Verification items for the finished model (mm, model axes). A direction names the side the tool comes from. Coordinates: 2 decimals unless noted, no trailing zeros. Loops run counter-clockwise (first coordinate to the right, second up) from the corner with the lowest first, then second, coordinate; pieces in that order, holes last. Notation, with made-up numbers: (79, 89.5) -> (95, 89.5) arc R19 ccw to (95, 106.5) -> close; hole circle Ø4 at (27, 60.5). An arc over 180 degrees is marked (long way). Write item = value, one per line.
```python
from build123d import *

# Parameters (mm, degrees)
BOSS_EXTRUDE1_DEPTH = 5.2832
SKETCH2_W           = 101.6
SKETCH2_H           = 14.351
BOSS_EXTRUDE2_DEPTH = 5.2832
CHAMFER1_SIZE       = 12.7
CHAMFER1_SIZE_2     = 3.81
CHAMFER2_SIZE       = 12.7
CHAMFER2_SIZE2      = 3.81
CHAMFER3_SIZE       = 3.81
CHAMFER3_SIZE_2     = 12.7


with BuildPart() as part:
    # Sketch1 → Boss-Extrude1 (new body)
    with BuildSketch(Plane(origin=(0, 0, 0), x_dir=(1, 0, 0), z_dir=(0, 1, 0))):
        Polygon((0, 0), (152.4, 0), (144.78, 68.834), (43.18, 68.834), align=None)
    extrude(amount=BOSS_EXTRUDE1_DEPTH)

    # Sketch2 → Boss-Extrude2 (add)
    with BuildSketch(Plane(origin=(0, 0, 0), x_dir=(1, 0, 0), z_dir=(0, 1, 0))):
        with Locations((76.2, -7.1755)):
            Rectangle(SKETCH2_W, SKETCH2_H)
    extrude(amount=BOSS_EXTRUDE2_DEPTH)

    # Chamfer1
    # the kernel refuses this chamfer: 12.7, 3.81 mm, written as the material it takes off along each edge
    with BuildSketch(Plane(origin=(60.699541801, 0, -96.762210753), x_dir=(0.8470671798621036, -0.011069119507992343, 0.531370555633054), z_dir=(-0.5314031118215187, 0, 0.8471190782566561))) as chamfer1_piece_1:
        Polygon((CHAMFER1_SIZE * 0.99993873542, CHAMFER1_SIZE * 0.011069119508), (-CHAMFER1_SIZE_2 * 0.011069119508, CHAMFER1_SIZE_2 * 0.99993873542), (0, 0), align=None)
    extrude(amount=147.193499363, mode=Mode.SUBTRACT)
    with BuildSketch(Plane(origin=(60.699541801, 5.2832, -96.762210753), x_dir=(0.8470671798621036, 0.01106911950799233, 0.531370555633054), z_dir=(-0.5314031118215187, 0, 0.8471190782566561))) as chamfer1_piece_2:
        Polygon((CHAMFER1_SIZE * 0.99993873542, -CHAMFER1_SIZE * 0.011069119508), (-CHAMFER1_SIZE_2 * 0.011069119508, -CHAMFER1_SIZE_2 * 0.99993873542), (0, 0), align=None)
    extrude(amount=147.193499363, mode=Mode.SUBTRACT)

    # Chamfer2
    chamfer2_edges = [part.edges().sort_by_distance(p)[0] for p in [
        (148.59, 0, -34.417),
    ]]
    chamfer2_side = [part.faces().sort_by_distance(p)[0] for p in [
        (89.414881318, 0, -25.614395123),
    ]]
    chamfer(chamfer2_edges, length=CHAMFER2_SIZE, length2=CHAMFER2_SIZE2, reference=chamfer2_side[0])

    # Chamfer3
    # the kernel refuses this chamfer: 12.7, 3.81 mm, written as the material it takes off along each edge
    with BuildSketch(Plane(origin=(156.027485672, 5.2832, 32.768287237), x_dir=(0.12133658482182727, -0.9925205348140393, -0.013432094260718893), z_dir=(-0.1100289719975825, 0, -0.9939283803781614))) as chamfer3_piece_1:
        Polygon((CHAMFER3_SIZE * 0.992520534814, CHAMFER3_SIZE * 0.122077794756), (-CHAMFER3_SIZE_2 * 0.122077794756, CHAMFER3_SIZE_2 * 0.992520534814), (0, 0), align=None)
    extrude(amount=135.191405264, mode=Mode.SUBTRACT)


solid = part.part
```
1) Sectioned sample at B-B, the plane z = -55.5. Record the cut outline in (x, y), plus the area to 3 significant figures.
Ans:
outline = (39.41, 2.64) -> (49.81, 0) -> (133.48, 0) -> (142.34, 2.64) -> (133.48, 5.28) -> (49.81, 5.28) -> close
area = 493 mm2
2) Depth check by flat-ended pin: pin 1 Ø1.6 at (y, z) = (3.5, 7) entering from +X; pin 2 Ø1.6 at (y, z) = (1.5, 10.5) entering from -X; pin 3 Ø1 at (x, z) = (23.5, -30.5) entering from +Y. Enter the tip coordinate at first touch or a pass-through.
Ans:
pin_1 = 127
pin_2 = 25.4
pin_3 = 2.73
3) Material ranges on line 1 (X direction, y = 0.6, z = 7.5); line 2 (Z direction, x = 128, y = 2.3); line 3 (Y direction, x = 138.5, z = -61.5), recorded low to high.
Ans:
line_1 = 25.4 to 127
line_2 = -68.83 to 0
line_3 = 1.7 to 3.59
4) Tool access check on faces 1 (the face through (17, 3, 0)), 2 (the face through (135, 3, 0)), 3 (the face through (90, 5.283, -28)). Record the directions out of +Z, -Z, +X, -X, +Y, -Y that give a thin tool (end or side, any length) a straight path to the whole face; none if there is none.
Ans:
face_1 = +Z, -X, +Y, -Y
face_2 = +Z, +X, +Y, -Y
face_3 = +Z, -Z, +X, -X, +Y
5) Sectioned sample at C-C, the plane x = 129.5. Record the cut outline in (y, z), plus the area to 3 significant figures.
Ans:
outline = (0, -68.83) -> (5.28, -68.83) -> (5.28, 0) -> (0, 0) -> close
area = 364 mm2
6) Sectioned sample at A-A, the plane y = 1.4. Record the cut outline in (x, z).
Ans:
outline = (9.48, 0) -> (52.66, -68.83) -> (136.7, -68.83) -> (144.32, 0) -> (127, 0) -> (127, 14.35) -> (25.4, 14.35) -> (25.4, 0) -> close
7) Sectioned sample at D-D, the plane z = -2.5. Record the cut outline in (x, y), plus the area to 3 significant figures.
Ans:
outline = (6.17, 2.64) -> (16.56, 0) -> (139.35, 0) -> (148.2, 2.64) -> (139.35, 5.28) -> (16.56, 5.28) -> close
area = 700 mm2
